Autodesk Fusion 360 part; units mm, degrees
sketch "Panel" plane through (0, 0, 0) normal (0, 1, 0) x (1, 0, 0)
  line L0 (250, -18) -> (250, -13)
  circle A0 centre (175, -148) radius 14
  line L1 (-140, -125) -> (-118, -171) construction
  circle A1 centre (-108, -148) radius 2.5
  circle A2 centre (152.5, -63) radius 2
  line L2 (140, -80) -> (140, -13) construction
  line L3 (-140, -125) -> (-140, -171)
  line L4 (123.1713, -63) -> (203.1713, -63) construction
  line L5 (-118, -125) -> (-140, -171) construction
  line L6 (250, -13) -> (-250, -13)
  line L7 (250, -213) -> (250, -13)
  circle A3 centre (100, -148) radius 14
  circle A4 centre (-150, -148) radius 2.5
  line L8 (-118, -171) -> (-118, -125)
  circle A5 centre (-50, -148) radius 14
  line L9 (-250, -213) -> (250, -213)
  line L10 (-250, -13) -> (-250, -213)
  line L11 (250, -13) -> (-250, -13)
  circle A6 centre (225, -53) radius 2.25
  line L12 (225, -213) -> (225, -13) construction
  line L13 (-140, -171) -> (-118, -171)
  line L14 (-118, -125) -> (-140, -125)
  line L15 (250, -148) -> (-250, -148) construction
  line L16 (-225, -213) -> (-225, -13) construction
  circle A7 centre (225, -173) radius 2.25
  circle A8 centre (-225, -53) radius 2.25
  circle A9 centre (-225, -173) radius 2.25
  circle A10 centre (126.8597, -63) radius 2
  line L17 (146.25, -57.25) -> (133.75, -57.25)
  line L18 (133.75, -57.25) -> (133.75, -68.75)
  line L19 (133.75, -68.75) -> (146.25, -68.75)
  line L20 (146.25, -68.75) -> (146.25, -57.25)
  line L21 (146.25, -57.25) -> (133.75, -68.75) construction
  line L22 (133.75, -57.25) -> (146.25, -68.75) construction
  point P0 (189, -148)
  point P1 (-152.5, -148)
  point P2 (-129, -148)
  point P3 (140, -63)
  dimension "d1" = 500
  dimension "d2" = 200
  dimension "d3" = 28
  dimension "d4" = 28
  dimension "d5" = 28
  dimension "d6" = 150
  dimension "d7" = 46
  dimension "d8" = 22
  dimension "d9" = 5
  dimension "d10" = 5
  dimension "d11" = 21
  dimension "d12" = 21
  dimension "d13" = 100
  dimension "d14" = 75
  dimension "d15" = 25
  dimension "d16" = 25
  dimension "d17" = 4.5
  dimension "d18" = 40
  dimension "d25" = 110
  dimension "d28" = 4
  dimension "d30" = 12.5
  dimension "d32" = 50
  dimension "d34" = 13
  dimension "d35" = 75
  dimension "d36" = 250
  dimension "d37" = 65
  dimension "d38" = 4.5
  dimension "d39" = 4.5
  dimension "d40" = 4.5
  dimension "d41" = 40
  dimension "d42" = 40
  dimension "d43" = 40
  dimension "d44" = 4
  dimension "d45" = 12.5
extrude "Extrude1" add sketch "Panel" along normal blind 3
equation "d4 = d3"
equation "d5 = d3"
equation "d6 = d140 * 2"
equation "d12 = d124"
equation "d18 = d41"
equation "d22 = d163"
equation "d36 = d1 / 2"
equation "d38 = d17"
equation "d39 = d17"
equation "d40 = d17"
equation "d42 = d41"
equation "d43 = d41"
equation "d44 = d28"
Model file for the job. Use its own axes, mm. Coordinates: 2 decimals unless noted, no trailing zeros. Order: outer loops, then holes, each group sorted by start corner. A loop starts at its lowest first (then second) coordinate and runs counter-clockwise, first axis right, second up. Notation, with made-up numbers: M 31,34.25 L 50,34.25 A16 cw 50,62.25 Z; hole C 5,63.25 d7. An arc over 180 degrees is marked long. Answer as CSV lines item,"result".
(1) Band-saw the part on A-A, the plane y = 0.55. State how many separate pieces and enclosed holes the cut face has, then the cut area to 3 significant figures.
Geometry says:
separate pieces,"1"
enclosed holes,"13"
area,"96,900 mm2"
(2) Band-saw the part on B-B, the plane x = 175. List the corners of the cut face in (y, z), then the cut area to 3 significant figures.
Geometry says:
outline,"M 0,13 L 3,13 L 3,134 L 0,134 Z; M 0,162 L 3,162 L 3,213 L 0,213 Z"
area,"516 mm2"
(3) Pull direction X, two halves, no side cores. Call faces 1 (the flat face through (-3, 0, 112)), 2 (the cylindrical face through (164.68, 1.48, 157.46)): +X half, -X half, draft (parallel to the pull), parting line (faces both ways), or undercut.
Geometry says:
face 1,"draft"
face 2,"undercut"
(4) Band-saw the part on C-C, the plane x = -47. List the corners of the cut face in (y, z).
Geometry says:
outline,"M 0,13 L 3,13 L 3,134.33 L 0,134.33 Z; M 0,161.67 L 3,161.67 L 3,213 L 0,213 Z"
(5) Wall check: line 1 along X through (y, z) = (1.3, 53); line 2 along Z through (x, y) = (-225, 1.65); line 3 along Z through (x, y) = (-133.5, 0.25). Give the ranges that are in metal, low to high.
Geometry says:
line 1,"x = -250 to -227.25, -222.75 to 222.75, 227.25 to 250"
line 2,"z = 13 to 50.75, 55.25 to 170.75, 175.25 to 213"
line 3,"z = 13 to 125, 171 to 213"
(6) Flat gauge pins, fed straight in: pin 1 (1 mm diameter, centred on x = 69.5, z = 67, fed in from -Y); pin 2 (4 mm diameter, centred on x = 225, z = 53, fed in from -Y). Where does each tip first touch, or does it go through?
Geometry says:
pin 1,"stops at y = 0"
pin 2,"passes through"
